Source: three-view drawing plus pictorial views. Frame: mm from the lowest corner of the part. Give positions to 0.01 mm unless a question says otherwise; leave off trailing zeros. Loops run counter-clockwise (first coordinate to the right, second up) from the corner with the lowest first, then second, coordinate; pieces in that order, holes last.
1. Draft query along X for the marked faces 1, 2 and 3. Return one class per face: +X half, -X half, draft (parallel to the pull), parting line (faces both ways), or undercut.
2. Material intervals for line 1 along Z through (x, y) = (90, 1.75) (1 decimal); line 2 along Z through (x, y) = (84, 1.5) (1 decimal); line 3 along X through (y, z) = (5, 85) (1 decimal), sorted ascending.
3. Section D-D, the plane x = 15. Output: boundary loops of the cut face in (y, z), then the cut area to 3 significant figures.
4. Section B-B, the plane z = 15. Output: boundary loops of the cut face in (x, y), then the cut area to 3 significant figures.
5. First-contact query: P1, Ø5, axis at x = 7.5, z = 15, coming from the +Y side; P2, Ø1.5, axis at x = 66, y = 5, coming from the +Z side; P3, Ø1.5, axis at y = 2.5, z = 87.5, coming from the -X side; P4, Ø4, axis at x = 64, z = 74, coming from the -Y side. Flat tips, straight axial feed; report the tip coordinate or a pass-through.
6. Section C-C, the plane y = 3.25. State how many separate pieces and enclosed holes the cut face has, then the cut area to 3 significant figures.
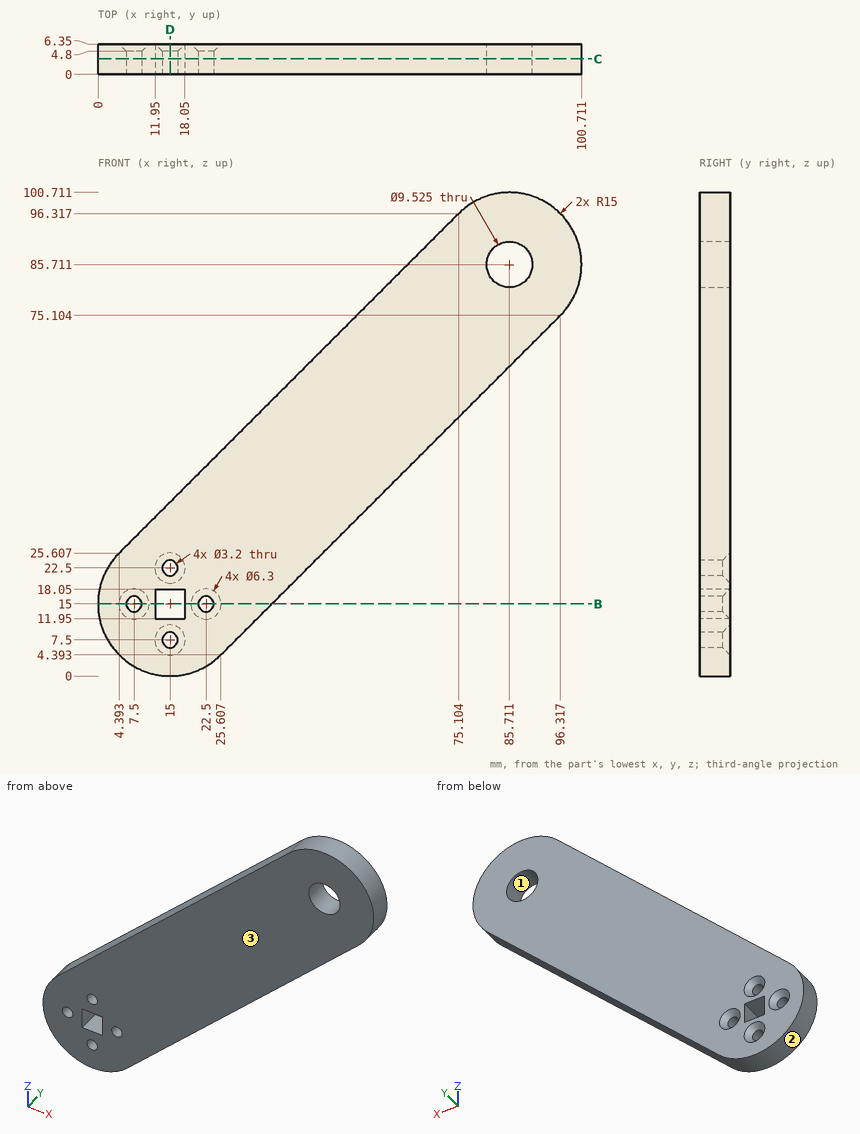
Answers below:
1. face 1: undercut
1. face 2: parting line
1. face 3: draft
2. line 1: z = 68.8 to 83.6, 87.8 to 100.1
2. line 2: z = 62.8 to 81.3, 90.2 to 100.6
2. line 3: x = 63.8 to 81, 90.4 to 100.7
3. outline: (0, 0) - (6.35, 0) - (6.35, 4.35) - (4.8, 5.9) - (0, 5.9) - close; (0, 9.1) - (4.8, 9.1) - (6.35, 10.65) - (6.35, 11.95) - (0, 11.95) - close; (0, 18.05) - (6.35, 18.05) - (6.35, 19.35) - (4.8, 20.9) - (0, 20.9) - close; (0, 24.1) - (4.8, 24.1) - (6.35, 25.65) - (6.35, 36.21) - (0, 36.21) - close
3. area: 146 mm2
4. outline: (0, 0) - (5.9, 0) - (5.9, 4.8) - (4.35, 6.35) - (0, 6.35) - close; (9.1, 0) - (11.95, 0) - (11.95, 6.35) - (10.65, 6.35) - (9.1, 4.8) - close; (18.05, 0) - (20.9, 0) - (20.9, 4.8) - (19.35, 6.35) - (18.05, 6.35) - close; (24.1, 0) - (36.21, 0) - (36.21, 6.35) - (25.65, 6.35) - (24.1, 4.8) - close
4. area: 146 mm2
5. P1: stops at y = 5.7
5. P2: stops at z = 87.96
5. P3: stops at x = 65.54
5. P4: stops at y = 0
6. separate pieces: 1
6. enclosed holes: 6
6. area: 3,570 mm2
